Geometry: final body of the model. Coordinates: model frame, mm. Round coordinates to 2 decimals unless told otherwise and drop trailing zeros. Loops run counter-clockwise (first coordinate to the right, second up) from the corner with the lowest first, then second, coordinate; pieces in that order, holes last. Notation, with made-up numbers: M -10,55.25 L 22,55.25 A27 ccw 22,89.25 Z; hole C 50.5,61.5 d2. An arc over 180 degrees is marked long. Return JSON: item names as keys, results as strings.
Autodesk Inventor part; units mm, degrees
ref_plane "YZ Plane" through (0, 0, 0) normal (1, 0, 0) x (0, 1, 0)
ref_plane "XZ Plane" through (0, 0, 0) normal (0, 1, 0) x (-1, 0, 0)
ref_plane "XY Plane" through (0, 0, 0) normal (0, 0, 1) x (1, 0, 0)
sketch "Skizze1" plane through (0, 0, 0) normal (0, 0, 1) x (1, 0, 0)
  line L0 (0, 0) -> (200, 0) construction
  line L1 (200, 0) -> (200, 40.1) construction
  line L2 (200, 40.1) -> (200, 41.6)
  line L3 (0, 0) -> (0, 70) construction
  line L4 (0, 70) -> (0, 71.5)
  arc A0 (100, 55.05) -> (0, 70) centre (0, -271.9232) ccw
  arc A1 (100, 55.05) -> (200, 40.1) centre (200, 382.0232) ccw
  arc A2 (100, 56.55) -> (0, 71.5) centre (0, -270.4232) ccw
  arc A3 (100, 56.55) -> (200, 41.6) centre (200, 383.5232) ccw
  line L5 (0, 71.5) -> (0, 101.5) construction
  line L6 (200, 41.6) -> (200, 78.6) construction
  line L7 (0, 101.5) -> (0, 103)
  line L8 (200, 78.6) -> (200, 80.1)
  line L9 (0, 103) -> (0, 133) construction
  line L10 (0, 133) -> (0, 134.5)
  line L11 (200, 80.1) -> (200, 122.4) construction
  line L12 (200, 122.4) -> (200, 123.9)
  arc A4 (100, 90.05) -> (200, 78.6) centre (200, 521.0062) ccw
  arc A5 (100, 91.55) -> (200, 80.1) centre (200, 522.5062) ccw
  arc A6 (100, 90.05) -> (0, 101.5) centre (0, -340.9062) ccw
  arc A7 (100, 91.55) -> (0, 103) centre (0, -339.4062) ccw
  arc A8 (100, 129.2) -> (200, 123.9) centre (200, 1069.9462) ccw
  arc A9 (100, 127.7) -> (0, 133) centre (0, -813.0462) ccw
  arc A10 (100, 127.7) -> (200, 122.4) centre (200, 1068.4462) ccw
  arc A11 (100, 129.2) -> (0, 134.5) centre (0, -811.5462) ccw
  line L13 (0, 0) -> (0, 190) construction
  line L14 (0, 190) -> (200, 190) construction
  line L15 (200, 190) -> (200, 191.5) construction
  line L16 (0, 190) -> (0, 191.5) construction
  line L17 (0, 191.5) -> (200, 191.5) construction
  line L18 (0, 0) -> (200, 0)
  point P0 (143.9749, 47.5506)
  point P1 (136.2206, 124.2462)
  point P2 (104.2284, 54.3303)
  dimension "d0" = 200
  dimension "d1" = 40.1
  dimension "d2" = 1.5
  dimension "d3" = 70
  dimension "d4" = 1.5
  dimension "d5" = 30
  dimension "d6" = 37
  dimension "d7" = 1.5
  dimension "d8" = 1.5
  dimension "d9" = 30
  dimension "d10" = 1.5
  dimension "d11" = 42.3
  dimension "d12" = 1.5
  dimension "d13" = 100
  dimension "d14" = 100
  dimension "d15" = 100
  dimension "d56" = 190
  dimension "d57" = 200
  dimension "d58" = 90
  dimension "d59" = 1.5
  dimension "d60" = 1.5
  dimension "d61" = 200
  dimension "d89" = 55.5
revolve "Umdrehung1" add sketch "Skizze1" angle 60 about axis through (0, 0, 0) along (-1, 0, 0) contours L7 A7 A5 L8 A4 A6 | L10 A11 A8 L12 A10 A9
sketch "Skizze3" plane through (0, 0, 0) normal (0, 0, 1) x (1, 0, 0)
  line L0 (200, 175.0528) -> (200, 191.5)
  line L1 (0, 191.5) -> (200, 191.5)
  arc A0 (100, 55.05) -> (0, 70) centre (0, -271.9232) ccw
  arc A1 (100, 55.05) -> (200, 40.1) centre (200, 382.0232) ccw
  line L2 (0, 70) -> (0, 191.5)
  line L3 (200, 191.5) -> (200, 40.1)
  point P0 (0, 0)
  point P1 (0, 0)
  point P2 (0, 0)
  point P3 (143.9749, 47.5506)
  point P4 (136.2206, 124.2462)
  point P5 (104.2284, 54.3303)
  point P6 (0, 0)
  dimension "d90" = 191.5
  dimension "d91" = 200
extrude "Extrusion1" add sketch "Skizze3" against normal blind 1.5
properties part number "Diffusoren mit Trennwand"
Q1. Material intervals for L1, parallel to Z at x = 144.5, y = 165; L2, parallel to Z at x = 25, y = 88.5; L3, parallel to Y at x = 97.5, z = -49, sorted ascending.
Determined:
{"L1": "z = -1.5 to 0", "L2": "z = -100.84 to -98.84, -51.3 to -48.24, -1.5 to 0", "L3": "y = 76.23 to 78.01, 118.21 to 119.83"}
Q2. Pin query (flat end, axial travel): pin 1 (10 mm diameter, centred on x = 24.5, z = -44, fed in from -Y); pin 2 (6 mm diameter, centred on x = 99, y = 165.5, fed in from -Z); pin 3 (12 mm diameter, centred on x = 121, y = 97, fed in from -Z). Return the tip coordinate at first contact, or that it passes through.
Determined:
{"pin 1": "stops at y = 88.09", "pin 2": "stops at z = -1.5", "pin 3": "stops at z = -88.92"}
Q3. Pull-direction query (Z, two-part tool) for faces 1 (the flat face through (99, 107, -1.5)), 2 (the flat face through (99.53, 64.24, -111.27)), 3 (the flat face through (99, 71, -1.5)), 4 (the flat face through (99, 117, 0)); classes: pulls with the +Z half, pulls with the -Z half, needs draft (parallel to the pull), parting line crosses it, or undercut.
Determined:
{"face 1": "undercut", "face 2": "pulls with the -Z half", "face 3": "undercut", "face 4": "pulls with the +Z half"}
Q4. Section query A-A (x = 124). Output: boundary loops of the cut face in (y, z), plus the area to 3 significant figures.
Determined:
{"outline": "M 42.59,-73.77 L 43.34,-75.06 A86.68 ccw 86.66,-1.5 L 125.45,-1.5 A125.46 cw 62.73,-108.65 L 63.48,-109.95 A126.96 ccw 126.95,-1.5 L 191.5,-1.5 L 191.5,0 L 48.65,0 L 48.65,-1.5 L 85.16,-1.5 A85.18 cw Z", "area": "543 mm^2"}
Q5. Section query C-C (x = 158). Output: boundary loops of the cut face in (y, z), plus the area to 3 significant figures.
Determined:
{"outline": "M 40.3,-69.8 L 41.05,-71.1 A82.1 ccw 82.08,-1.5 L 123.32,-1.5 A123.33 cw 61.67,-106.81 L 62.42,-108.11 A124.83 ccw 124.82,-1.5 L 191.5,-1.5 L 191.5,0 L 42.69,0 L 42.69,-1.5 L 80.58,-1.5 A80.6 cw Z", "area": "541 mm^2"}
Q6. Section query B-B (y = 172). Output: boundary loops of the cut face in (x, z).
Determined:
{"outline": "M 0,-1.5 L 200,-1.5 L 200,0 L 0,0 Z"}
